Part model, mm, in its own coordinate system. Face numbers are marked on the shaded views. Round coordinates to 2 decimals unless told otherwise and drop trailing zeros. Loops run counter-clockwise (first coordinate to the right, second up) from the corner with the lowest first, then second, coordinate; pieces in that order, holes last.
1) Probe line 1 (Y direction, x = 9.5, z = -2); line 2 (Y direction, x = 30, z = -2.5); line 3 (Y direction, x = 19, z = -12). List the from-to ranges inside material, lowest first.
2) Drop flat-ended pins along their axis: P1, Ø5, axis at x = 27.25, z = 0, coming from the -Y side; P2, Ø10, axis at y = 206.5, z = -13.5, coming from the +X side; P3, Ø5, axis at x = -29.5, z = -1, coming from the +Y side. Give the stop position or say it passes through.
3) Band-saw the part on B-B, the plane y = 244. Write the cut outline in (x, z), then the cut area to 3 significant figures.
4) Mould opens along Y. For the marked faces 1, 2 and 3 say: +Y half, -Y half, draft (parallel to the pull), parting line (faces both ways), or undercut.
5) Band-saw the part on A-A, the plane y = 31. Write the cut outline in (x, z), then the cut area to 3 significant figures.
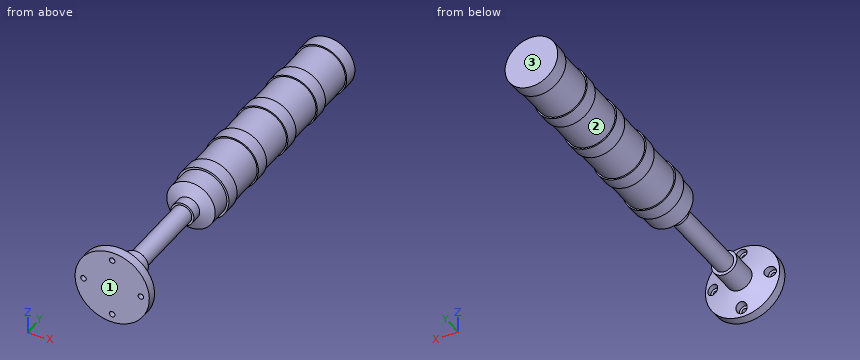
from build123d import *

# Parameters (mm, degrees)
SKETCH1_R           = 35.25
BOSS_EXTRUDE1_DEPTH = 9
SKETCH3_R           = 12
BOSS_EXTRUDE2_DEPTH = 26
SKETCH4_R           = 9
BOSS_EXTRUDE3_DEPTH = 80
SKETCH5_R           = 11
BOSS_EXTRUDE4_DEPTH = 10
SKETCH7_R           = 23
BOSS_EXTRUDE5_DEPTH = 20
SKETCH9_R           = 2.65
CUT_EXTRUDE1_DEPTH  = 20
CUT_EXTRUDE2_START  = 45
SKETCH11_R          = 5.25
CUT_EXTRUDE2_DEPTH  = 40


with BuildPart() as part:
    # Sketch1 → Boss-Extrude1 (new body)
    with BuildSketch(Plane(origin=(0, 0, 0), x_dir=(1, 0, 0), z_dir=(0, 1, 0))):
        with Locations(Location((0, 0, 0), (0, 0, 270))):
            Circle(SKETCH1_R)
    extrude(amount=BOSS_EXTRUDE1_DEPTH)

    # Sketch2 → Revolve1 (revolve)
    with BuildSketch(Plane.XY, mode=Mode.PRIVATE) as revolve1_sk:
        Polygon((0, 9), (0, 14.5), (12, 14.5), (35.25, 9), align=None)
    revolve(revolve1_sk.sketch.rotate(Axis((0, 9, 0), (0, 1, 0)), 90), axis=Axis((0, 9, 0), (0, 1, 0)))

    # Sketch3 → Boss-Extrude2 (add)
    with BuildSketch(Plane(origin=(0, 14.5, 0), x_dir=(1, 0, 0), z_dir=(0, 1, 0))):
        with Locations(Location((0, 0, 0), (0, 0, 90))):
            Circle(SKETCH3_R)
    extrude(amount=BOSS_EXTRUDE2_DEPTH)

    # Sketch4 → Boss-Extrude3 (add)
    with BuildSketch(Plane(origin=(0, 40.5, 0), x_dir=(1, 0, 0), z_dir=(0, 1, 0))):
        with Locations(Location((0, 0, 0), (0, 0, 270))):
            Circle(SKETCH4_R)
    extrude(amount=BOSS_EXTRUDE3_DEPTH)

    # Sketch5 → Boss-Extrude4 (add)
    with BuildSketch(Plane(origin=(0, 120.5, 0), x_dir=(1, 0, 0), z_dir=(0, 1, 0))):
        with Locations(Location((0, 0, 0), (0, 0, 270))):
            Circle(SKETCH5_R)
    extrude(amount=BOSS_EXTRUDE4_DEPTH)

    # Sketch6 → Revolve2 (revolve)
    with BuildSketch(Plane.XY, mode=Mode.PRIVATE) as revolve2_sk:
        Polygon((0, 130.5), (0, 135.5), (23, 135.5), (11, 130.5), align=None)
    revolve(revolve2_sk.sketch.rotate(Axis((0, 130.5, 0), (0, 1, 0)), 270), axis=Axis((0, 130.5, 0), (0, 1, 0)))

    # Sketch7 → Boss-Extrude5 (add)
    with BuildSketch(Plane(origin=(0, 135.5, 0), x_dir=(1, 0, 0), z_dir=(0, 1, 0))):
        with Locations(Location((0, 0, 0), (0, 0, 270))):
            Circle(SKETCH7_R)
    extrude(amount=BOSS_EXTRUDE5_DEPTH)

    # Sketch8 → Revolve6 (revolve)
    with BuildSketch(Plane.XY, mode=Mode.PRIVATE) as revolve6_sk:
        Polygon((-25, 155.5), (0, 155.5), (0, 372.060698134), (-25, 372.060698134), (-25, 358.060698134), (-23.75, 358.060698134), (-23.75, 321.420523601), (-25, 321.420523601), (-25, 307.420523601), (-23.75, 307.420523601), (-23.75, 270.780349067), (-25, 270.780349067), (-25, 256.780349067), (-23.75, 256.780349067), (-23.75, 220.140174534), (-25, 220.140174534), (-25, 206.140174534), (-23.75, 206.140174534), (-23.75, 169.5), (-25, 169.5), align=None)
    revolve(revolve6_sk.sketch.rotate(Axis((0, 155.5, 0), (0, 1, 0)), 270), axis=Axis((0, 155.5, 0), (0, 1, 0)))

    # Sketch9 → Cut-Extrude1 (cut)
    with BuildSketch(Plane.XZ):
        with Locations(Location((0, 27.25, 0), (0, 0, 270))):
            Circle(SKETCH9_R)
        with Locations(Location((27.25, 0, 0), (0, 0, 270))):
            Circle(SKETCH9_R)
        with Locations(Location((0, -27.25, 0), (0, 0, 270))):
            Circle(SKETCH9_R)
        with Locations(Location((-27.25, 0, 0), (0, 0, 270))):
            Circle(SKETCH9_R)
    extrude(amount=-CUT_EXTRUDE1_DEPTH, mode=Mode.SUBTRACT)

    # Sketch11 → Cut-Extrude2 (cut)
    with BuildSketch(Plane(origin=(0, 0, 0), x_dir=(1, 0, 0), z_dir=(0, 1, 0)).offset(CUT_EXTRUDE2_START)):
        with Locations(Location((0, 27.25, 0), (0, 0, 270))):
            Circle(SKETCH11_R)
        with Locations(Location((27.25, 0, 0), (0, 0, 270))):
            Circle(SKETCH11_R)
        with Locations(Location((0, -27.25, 0), (0, 0, 270))):
            Circle(SKETCH11_R)
        with Locations(Location((-27.25, 0, 0), (0, 0, 270))):
            Circle(SKETCH11_R)
    extrude(amount=-CUT_EXTRUDE2_DEPTH, mode=Mode.SUBTRACT)


solid = part.part
Reported:
1. line 1: y = 0 to 40.5, 120.5 to 372.06
1. line 2: y = 0 to 5
1. line 3: y = 0 to 12.02, 135.28 to 372.06
2. P1: stops at y = 155.5
2. P2: stops at x = 23.51
2. P3: stops at y = 5
3. outline: circle Ø47.5 at (0, 0)
3. area: 1,770 mm2
4. face 1: -Y half
4. face 2: undercut
4. face 3: +Y half
5. outline: circle Ø24 at (0, 0)
5. area: 452 mm2
